Geometry check sheet. Reference: the model listing, model coordinates, mm. A direction names the side the tool comes from. Coordinates: 2 decimals unless noted, no trailing zeros. Write each loop counter-clockwise with the first axis right and the second up, starting at its lowest first coordinate (ties: lowest second). Pieces come first, ordered by that corner, then holes.
from build123d import *

# Parameters (mm, degrees)
SKETCH1_R           = 10.5
SKETCH1_R_2         = 6
BOSS_EXTRUDE1_DEPTH = 57
SKETCH2_W           = 32
SKETCH2_H           = 32
SKETCH2_R           = 6
BOSS_EXTRUDE2_DEPTH = 6
SKETCH3_R           = 2.25
CUT_EXTRUDE1_DEPTH  = 62.326992426
CHAMFER1_SIZE       = 3
SKETCH5_R           = 3.75
CUT_EXTRUDE2_DEPTH  = 4.1


with BuildPart() as part:
    # Sketch1 → Boss-Extrude1 (new body)
    with BuildSketch(Plane(origin=(0, 0, 0), x_dir=(1, 0, 0), z_dir=(0, 1, 0))):
        with Locations(Location((0, 0, 0), (0, 0, 90))):
            Circle(SKETCH1_R)
        with Locations(Location((0, 0, 0), (0, 0, 90))):
            Circle(SKETCH1_R_2, mode=Mode.SUBTRACT)
    extrude(amount=BOSS_EXTRUDE1_DEPTH)

    # Sketch2 → Boss-Extrude2 (add)
    with BuildSketch(Plane(origin=(0, 0, 0), x_dir=(1, 0, 0), z_dir=(0, 1, 0))):
        Rectangle(SKETCH2_W, SKETCH2_H)
        with Locations(Location((0, 0, 0), (0, 0, 90))):
            Circle(SKETCH2_R, mode=Mode.SUBTRACT)
    extrude(amount=BOSS_EXTRUDE2_DEPTH)

    # Sketch3 → Cut-Extrude1 (cut, through all)
    with BuildSketch(Plane(origin=(0, 0, 0), x_dir=(1, 0, 0), z_dir=(0, 1, 0))):
        with Locations(Location((-11.313708499, 11.313708499, 0), (0, 0, 90))):
            Circle(SKETCH3_R)
        with Locations(Location((-11.313708499, -11.313708499, 0), (0, 0, 90))):
            Circle(SKETCH3_R)
        with Locations(Location((11.313708499, -11.313708499, 0), (0, 0, 90))):
            Circle(SKETCH3_R)
        with Locations(Location((11.313708499, 11.313708499, 0), (0, 0, 90))):
            Circle(SKETCH3_R)
    extrude(amount=CUT_EXTRUDE1_DEPTH, mode=Mode.SUBTRACT)

    # Chamfer1
    chamfer1_edges = [part.edges().sort_by_distance(p)[0] for p in [
        (16, 3, 16),
        (16, 3, -16),
        (-16, 3, -16),
        (-16, 3, 16),
    ]]
    chamfer(chamfer1_edges, length=CHAMFER1_SIZE)

    # Sketch5 → Cut-Extrude2 (cut)
    with BuildSketch(Plane.XZ):
        with Locations(Location((-11.313708499, 11.313708499, 0), (0, 0, 270))):
            Circle(SKETCH5_R)
        with Locations(Location((11.313708499, 11.313708499, 0), (0, 0, 270))):
            Circle(SKETCH5_R)
        with Locations(Location((11.313708499, -11.313708499, 0), (0, 0, 270))):
            Circle(SKETCH5_R)
        with Locations(Location((-11.313708499, -11.313708499, 0), (0, 0, 270))):
            Circle(SKETCH5_R)
    extrude(amount=-CUT_EXTRUDE2_DEPTH, mode=Mode.SUBTRACT)


solid = part.part
1. Thickness scan on line 1 along Y through (x, z) = (-10.5, -5); line 2 along X through (y, z) = (30, 4.5); line 3 along Z through (x, y) = (3, 51.5). Record the ranges inside material, lowest first.
Computed values:
line 1: y = 0 to 6
line 2: x = -9.49 to -3.97, 3.97 to 9.49
line 3: z = -10.06 to -5.2, 5.2 to 10.06
2. Gauge pin test, flat ends, axial feed: pin 1 Ø7 at (x, z) = (-11.31, -11.31) entering from -Y; pin 2 Ø8.5 at (x, z) = (11.31, 11.31) entering from +Y; pin 3 Ø1 at (x, y) = (5, 20.5) entering from -Z; pin 4 Ø2 at (x, z) = (-11.5, -10.5) entering from -Y. Record the tip position at first contact, or that the pin passes through.
Computed values:
pin 1: stops at y = 4.1
pin 2: stops at y = 6
pin 3: stops at z = -9.49
pin 4: passes through
3. Sectioned sample at A-A, the plane x = 0. Record the boundary of the cut face in (y, z), and give its area (3 significant figures).
Computed values:
outline: (0, -16) - (6, -16) - (6, -10.5) - (57, -10.5) - (57, -6) - (0, -6) - close; (0, 6) - (57, 6) - (57, 10.5) - (6, 10.5) - (6, 16) - (0, 16) - close
area: 579 mm2
4. Draft check along X on faces 4 (the flat face through (-11.3, 4.1, 8.9)), 5 (the flat face through (-16, 3, 0)), 6 (the flat face through (15, 3, 14)). Enter one of: released by +X, released by -X, zero draft, split by the parting line, or undercut.
Computed values:
face 4: undercut
face 5: released by -X
face 6: released by +X
5. Sectioned sample at C-C, the plane x = 12. Record the boundary of the cut face in (y, z).
Computed values:
outline: (0, -16) - (6, -16) - (6, -13.46) - (4.1, -13.46) - (4.1, -15) - (0, -15) - close; (0, -7.63) - (4.1, -7.63) - (4.1, -9.17) - (6, -9.17) - (6, 9.17) - (4.1, 9.17) - (4.1, 7.63) - (0, 7.63) - close; (0, 15) - (4.1, 15) - (4.1, 13.46) - (6, 13.46) - (6, 16) - (0, 16) - close
6. Sectioned sample at D-D, the plane y = 50. Record the boundary of the cut face in (x, z), and give its area (3 significant figures).
Computed values:
outline: circle Ø21 at (0, 0); hole circle Ø12 at (0, 0)
area: 233 mm2
7. Sectioned sample at B-B, the plane z = 0. Record the boundary of the cut face in (x, y), and give its area (3 significant figures).
Computed values:
outline: (-16, 0) - (-6, 0) - (-6, 57) - (-10.5, 57) - (-10.5, 6) - (-16, 6) - close; (6, 0) - (16, 0) - (16, 6) - (10.5, 6) - (10.5, 57) - (6, 57) - close
area: 579 mm2
8. Access from +Z, -Z, +X, -X, +Y, -Y to the whole of each face (thin tool, end or side, straight path). Record for faces 1 (the flat face through (11.4, 4.1, 8.9)), 2 (the flat face through (-14, 3, -15)), 3 (the cylindrical face through (-3.2, 31.1, -10)).
Computed values:
face 1: -Y
face 2: -Z, -X, +Y, -Y
face 3: +Y
